Check sheet for the drawn part. Datum: minimum x, y, z corner. Units: mm. Round coordinates to 2 decimals unless told otherwise and drop trailing zeros. Write each loop counter-clockwise with the first axis right and the second up, starting at its lowest first coordinate (ties: lowest second). Pieces come first, ordered by that corner, then holes. Notation, with made-up numbers: M 44.25,41 L 66.25,41 A21 cw 66.25,79 Z; hole C 78,20 d11. An arc over 180 degrees is marked long. Answer in a Markdown table with one row per item. Add a question column.
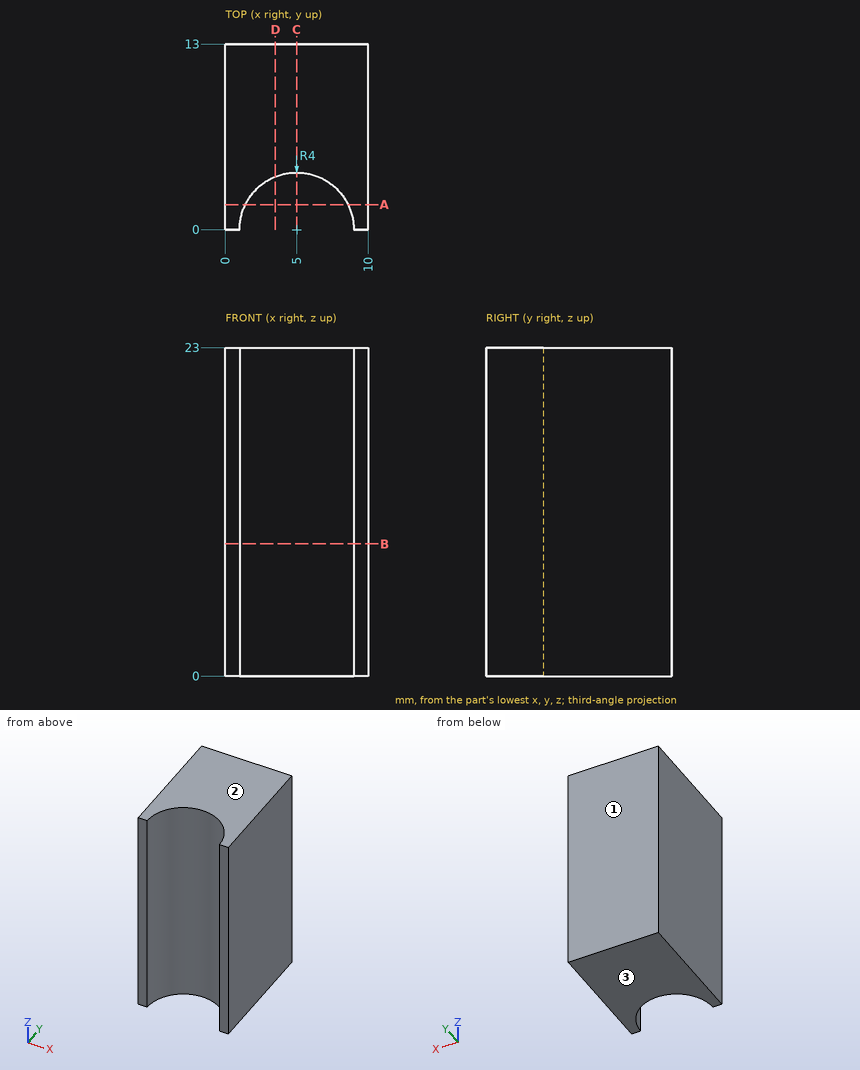
Item 1: Section check B-B, the plane z = 9.25. Record the boundary of the cut face in (x, y), and give its area (3 significant figures).
Item 2: Gauge pin test, flat ends, axial feed: pin 1 Ø4 at (x, y) = (9, 9.5) entering from -Z; pin 2 Ø2 at (x, z) = (3, 11.5) entering from -Y. Record the tip position at first contact, or that the pin passes through.
Item 3: Section check C-C, the plane x = 5. Record the boundary of the cut face in (y, z).
Item 4: Section check D-D, the plane x = 3.5. Record the boundary of the cut face in (y, z), and give its area (3 significant figures).
Item 5: Mould release check, pull along Z, two halves, no side actions. Record for the marked faces 1, 2 and 3: +Z half, -Z half, draft (parallel to the pull), parting line (faces both ways), or undercut.
Item 6: Section check A-A, the plane y = 1.75. Record the boundary of the cut face in (x, z), and give its area (3 significant figures).
Item 7: Scan lines: probe 1 along Y at (x, z) = (5, 15); probe 2 along Y at (x, z) = (3.25, 5); probe 3 along X at (y, z) = (1.5, 2.25). Record each from-to range of solid material in increasing order. Write a range as from..to.
Result sheet:
| question | item | result |
|---|---|---|
| 1 | outline | M 0,0 L 1,0 A4 cw 9,0 L 10,0 L 10,13 L 0,13 Z |
| 1 | area | 105 mm^2 |
| 2 | pin 1 | stops at z = 0 |
| 2 | pin 2 | stops at y = 2.65 |
| 3 | outline | M 4,0 L 13,0 L 13,23 L 4,23 Z |
| 4 | outline | M 3.71,0 L 13,0 L 13,23 L 3.71,23 Z |
| 4 | area | 214 mm^2 |
| 5 | face 1 | draft |
| 5 | face 2 | +Z half |
| 5 | face 3 | -Z half |
| 6 | outline | M 0,0 L 1.4,0 L 1.4,23 L 0,23 Z; M 8.6,0 L 10,0 L 10,23 L 8.6,23 Z |
| 6 | area | 64.5 mm^2 |
| 7 | probe 1 | y = 4..13 |
| 7 | probe 2 | y = 3.6..13 |
| 7 | probe 3 | x = 0..1.29, 8.71..10 |
